Source: CAD feature listing. Evaluate the final solid. Frame: model axes, mm. A direction names the side the tool comes from. Give positions to 0.01 mm unless a question says otherwise; leave off trailing zeros. Write each loop counter-clockwise with the first axis right and the second up, starting at its lowest first coordinate (ties: lowest second). Pieces come first, ordered by that corner, then holes. Notation, with made-up numbers: (84.25, 29.5) -> (99.25, 29.5) arc R30 ccw to (99.25, 52.5) -> close; hole circle Ø7 at (42.5, -34.5). An arc over 180 degrees is marked (long way). Use one line per item in the form item = value. Start each with the question number.
(1) Material intervals for line 1 along X through (y, z) = (4.75, -1.5); line 2 along Z through (x, y) = (-51.5, 6.5); line 3 along Z through (x, y) = (20.5, 4.5), sorted ascending. Write a range as from..to.
(2) Cut plane A-A, the plane y = 7. Output: boundary loops of the cut face in (x, z).
(3) Set-up query: faces 4 (the face through (-28.574, 3.944, 21.34)), 5 (the face through (-40.61, 5.04, 63.63)), 6 (the face through (25.61, 5.04, -0.62)), 7 (the face through (22.245, 5.042, -4.97)), 8 (the face through (-45.019, 3.055, 65.425)). Return all of +Z, -Z, +X, -X, +Y, -Y with unobstructed straight access to the full face (end or side cutting, diameter ignored); none if empty.
(4) Cut plane D-D, the plane x = -5.5. Output: boundary loops of the cut face in (y, z), and give its area (3 significant figures).
(5) Cut plane C-C, the plane z = 30.5. Output: boundary loops of the cut face in (x, y) (3 decimals).
(6) Draft query along X for faces 1 (the face through (-42.3, 3.9, 67.6)), 2 (the face through (24.799, 4.056, 1.614)), 3 (the face through (25, 2, -4)). Return one class per face: pulls with the +X half, pulls with the -X half, needs draft (parallel to the pull), parting line crosses it, or undercut.
(7) Cut plane B-B, the plane x = -49. Output: boundary loops of the cut face in (y, z) (3 decimals).
(8) First-contact query: P1, Ø1.5, axis at x = -19, y = 6, coming from the -Z side; P2, Ø1, axis at x = 2.5, y = 1, coming from the +Z side. Flat tips, straight axial feed; report the tip coordinate or a pass-through.
from build123d import *

# Parameters (mm, degrees)
SKETCH1_R           = 2.75
BOSS_EXTRUDE1_DEPTH = 8
CUT_EXTRUDE1_DEPTH  = 6
CUT_EXTRUDE2_DEPTH  = 30.169438933
BOSS_EXTRUDE2_START = -8
SKETCH4_R           = 2.75
BOSS_EXTRUDE2_DEPTH = 8
CUT_EXTRUDE3_DEPTH  = 6
FILLET1_R           = 5


with BuildPart() as part:
    # Sketch1 → Boss-Extrude1 (new body)
    with BuildSketch(Plane(origin=(0, 0, 0), x_dir=(1, 0, 0), z_dir=(0, 1, 0))):
        with BuildLine():
            Line((-7.712527276, 6.5), (22.287472724, 6.5))
            ThreePointArc((22.287472724, 6.5), (27.287472724, 1.5), (22.287472724, -3.5))
            Line((22.287472724, -3.5), (-7.712527276, -3.5))
            ThreePointArc((-7.712527276, -3.5), (-12.712527276, 1.5), (-7.712527276, 6.5))
        make_face()
        with Locations(Location((22.287472724, 1.5, 0), (0, 0, 270))):
            Circle(SKETCH1_R, mode=Mode.SUBTRACT)
    extrude(amount=BOSS_EXTRUDE1_DEPTH)

    # Sketch2 → Cut-Extrude1 (cut)
    with BuildSketch(Plane(origin=(0, 8, 0), x_dir=(1, 0, 0), z_dir=(0, 1, 0))):
        Polygon((20.58345093, 3.658427605), (23.991494517, -0.658427605), (33.922344634, 7.181717223), (30.514301047, 11.498572433), align=None)
    extrude(amount=-CUT_EXTRUDE1_DEPTH, mode=Mode.SUBTRACT)

    # Sketch3 → Cut-Extrude2 (cut, through all)
    with BuildSketch(Plane(origin=(0, 8, 0), x_dir=(1, 0, 0), z_dir=(0, 1, 0))):
        Polygon((19.607061, -5.712417018), (21.868852578, -8.577353017), (34.080402114, 1.063343984), (31.818610536, 3.928279983), align=None)
    extrude(amount=-CUT_EXTRUDE2_DEPTH, mode=Mode.SUBTRACT)

    # Sketch4 → Boss-Extrude2 (add)
    with BuildSketch(Plane(origin=(0, 8, 0), x_dir=(1, 0, 0), z_dir=(0, 1, 0)).offset(BOSS_EXTRUDE2_START)):
        with BuildLine():
            Line((-4.614305833, -2.424413828), (-54.336629031, -41.678879507))
            Line((-54.336629031, -41.678879507), (-40.041435295, -59.786124909))
            ThreePointArc((-40.041435295, -59.786124909), (-40.86762768, -66.808760179), (-47.89026295, -65.982567794))
            Line((-47.89026295, -65.982567794), (-65.28367813, -43.950908565))
            ThreePointArc((-65.28367813, -43.950908565), (-66.325017324, -40.268480884), (-64.457485745, -36.928273294))
            Line((-64.457485745, -36.928273294), (-10.810748719, 5.424413828))
            ThreePointArc((-10.810748719, 5.424413828), (-3.788113448, 4.598221443), (-4.614305833, -2.424413828))
        make_face()
        with Locations(Location((-43.965849122, -62.884346351, 0), (0, 0, 270))):
            Circle(SKETCH4_R, mode=Mode.SUBTRACT)
    extrude(amount=BOSS_EXTRUDE2_DEPTH)

    # Sketch5 → Cut-Extrude3 (cut)
    with BuildSketch(Plane(origin=(0, 8, 0), x_dir=(1, 0, 0), z_dir=(0, 1, 0))):
        Polygon((-45.754712001, -60.795693771), (-42.176986244, -64.972998932), (-32.718063171, -56.871739527), (-36.295788929, -52.694434367), align=None)
    extrude(amount=-CUT_EXTRUDE3_DEPTH, mode=Mode.SUBTRACT)

    # Fillet1
    fillet1_edges = [part.edges().sort_by_distance(p)[0] for p in [
        (-5.976714985, 4, 3.5),
        (-54.336629031, 4, 41.678879507),
    ]]
    fillet(fillet1_edges, radius=FILLET1_R)


solid = part.part
Geometry says:
q1.line_1 = -15.78..19.54, 26.73..27.29
q1.line_2 = 26.7..39.77, 45.24..61.41
q1.line_3 = -6.5..-3.59, 0.59..3.5
q2.outline = (-65.28, 43.95) arc R5 ccw to (-64.46, 36.93) -> (-10.81, -5.42) arc R5 ccw to (-7.71, -6.5) -> (22.29, -6.5) arc R5 ccw to (23.86, -6.25) -> (20.58, -3.66) arc R2.75 cw to (23.99, 0.66) -> (27.27, -1.93) arc R5 ccw to (27.12, -0.22) -> (22.41, 3.5) arc R5 ccw to (22.29, 3.5) -> (-4.24, 3.5) arc R5 cw to (-7.34, 4.58) -> (-50.41, 38.58) arc R5 cw to (-51.24, 45.6) -> (-41.87, 57.47) -> (-45.75, 60.8) arc R2.75 cw to (-42.18, 64.97) -> (-39.01, 62.26) arc R5 ccw to (-47.89, 65.98) -> close
q3.face_4 = +X, +Y, -Y
q3.face_5 = +Y
q3.face_6 = -Z, +Y
q3.face_7 = +X, +Y
q3.face_8 = +Y, -Y
q4.outline = (0, -6.5) -> (8, -6.5) -> (8, 3.66) -> (0, 3.66) -> close
q4.area = 81.3 mm^2
q5.outline = (-56.315, 0) -> (-40.177, 0) -> (-40.177, 8) -> (-56.315, 8) -> close
q6.face_1 = parting line crosses it
q6.face_2 = pulls with the +X half
q6.face_3 = undercut
q7.outline = (0, 24.725) -> (8, 24.725) -> (8, 37.466) -> (0, 37.466) -> close; (0, 48.439) -> (8, 48.439) -> (8, 64.577) -> (0, 64.577) -> close
q8.P1 = 0.45
q8.P2 = 3.5
